from build123d import *

# Parameters (mm, degrees)
SKETCH1_R           = 1.2
BOSS_EXTRUDE1_DEPTH = 4
FILLET1_R           = 5


with BuildPart() as part:
    # Sketch1 → Boss-Extrude1 (new body)
    with BuildSketch(Plane.XY):
        with BuildLine():
            Line((0, 0), (38.39, 0))
            Line((38.39, 0), (38.39, 20))
            Line((38.39, 20), (20, 20))
            ThreePointArc((20, 20), (0, 20), (0, 0))
        make_face()
        Polygon((3.79, 3.79), (3.79, 7.5), (2.59, 7.5), (2.59, 12.5), (3.79, 12.5), (3.79, 16.21), (26.39, 16.21), (26.39, 3.79), align=None, mode=Mode.SUBTRACT)
        with Locations((10, 20.176067812)):
            Circle(SKETCH1_R, mode=Mode.SUBTRACT)
        with Locations((32.39, 10)):
            Circle(SKETCH1_R, mode=Mode.SUBTRACT)
    extrude(amount=BOSS_EXTRUDE1_DEPTH)

    # Fillet1
    fillet1_edges = [part.edges().sort_by_distance(p)[0] for p in [
        (38.39, 20, 2),
        (38.39, 0, 2),
        (0, 0, 2),
        (20, 20, 2),
    ]]
    fillet(fillet1_edges, radius=FILLET1_R)


solid = part.part
Can you work these out from the model? Positions are in its coordinate system, mm. A direction names the side the tool comes from. Coordinates: 2 decimals unless noted, no trailing zeros. Write each loop counter-clockwise with the first axis right and the second up, starting at its lowest first coordinate (ties: lowest second). Pieces come first, ordered by that corner, then holes. Notation, with made-up numbers: (89.5, 8) -> (110.5, 8) arc R10 cw to (110.5, 12) -> close; hole circle Ø6 at (-9.75, 78). An arc over 180 degrees is marked (long way). Write each question's results on one line, items separated by ' | '. Start each with the question number.
Item 1: If we section it at A-A, the plane x = 32.39: Write out the boundary of the cut face in (y, z), and give its area (3 significant figures).
Item 2: If we section it at D-D, the plane y = 13.75: Write out the boundary of the cut face in (x, z).
Item 3: Please list where these lines run through material, in increasing order: probe 1 along Y at (x, z) = (10, 0.85); probe 2 along Y at (x, z) = (32.39, 2.8); probe 3 along Y at (x, z) = (30, 2.9).
Item 4: If we section it at B-B, the plane y = 10: Write out the boundary of the cut face in (x, z), and give its area (3 significant figures).
Item 5: On a 3-axis mill with a long thin cutter (end or side, diameter ignored), from which of +Z, -Z, +X, -X, +Y, -Y can I reach the whole of each face in a straight line? I mean faces 4 (the flat face through (17, 18, 4)), 5 (the flat face through (3.79, 6, 2)). Say none if no direction works.
Item 6: I'm going to push flat-ended pins straight in: P1, Ø1, axis at x = 6, z = 2.5, coming from the +Y side; P2, Ø1, axis at x = 3.5, z = 1.5, coming from the +Y side. Where does each tip first touch, or does it pass through?
Item 7: Thinking about a two-plate mould opening in Y: for faces 1 (the flat face through (28, 20, 2)), 2 (the cylindrical face through (0.677, 20.634, 1.972)), 3 (the flat face through (15, 16.21, 2)), which applies, released by +Y, released by -Y, zero draft, split by the parting line, or undercut?
Item 8: If we section it at C-C, the plane x = 10: Write out the boundary of the cut face in (y, z), and give its area (3 significant figures).
Answer block:
1) outline: (0, 0) -> (8.8, 0) -> (8.8, 4) -> (0, 4) -> close; (11.2, 0) -> (20, 0) -> (20, 4) -> (11.2, 4) -> close | area: 70.4 mm²
2) outline: (-3.64, 0) -> (3.79, 0) -> (3.79, 4) -> (-3.64, 4) -> close; (26.39, 0) -> (38.39, 0) -> (38.39, 4) -> (26.39, 4) -> close
3) probe 1: 0 to 3.79, 16.21 to 18.98, 21.38 to 24.14 | probe 2: 0 to 8.8, 11.2 to 20 | probe 3: 0 to 20
4) outline: (-4.14, 0) -> (2.59, 0) -> (2.59, 4) -> (-4.14, 4) -> close; (26.39, 0) -> (31.19, 0) -> (31.19, 4) -> (26.39, 4) -> close; (33.59, 0) -> (38.39, 0) -> (38.39, 4) -> (33.59, 4) -> close | area: 65.3 mm²
5) face 4: +Z, +X, -X, +Y, -Y | face 5: +Z, -Z
6) P1: y = 23.7 | P2: y = 22.81
7) face 1: released by +Y | face 2: split by the parting line | face 3: undercut
8) outline: (0, 0) -> (3.79, 0) -> (3.79, 4) -> (0, 4) -> close; (16.21, 0) -> (18.98, 0) -> (18.98, 4) -> (16.21, 4) -> close; (21.38, 0) -> (24.14, 0) -> (24.14, 4) -> (21.38, 4) -> close | area: 37.3 mm²
